The listing builds one solid part. Answer for the finished solid, in the listing's coordinates (mm). A direction names the side the tool comes from. Round coordinates to 2 decimals unless told otherwise and drop trailing zeros. Loops run counter-clockwise (first coordinate to the right, second up) from the corner with the lowest first, then second, coordinate; pieces in that order, holes last. Notation, with made-up numbers: (-33.75, -10) -> (9.25, -10) arc R19 ccw to (9.25, 10) -> close; hole circle Ø8 at (-5.5, -22.5). An arc over 180 degrees is marked (long way). One line per question, with ' | ' between items.
from build123d import *

# Parameters (mm, degrees)
F0_R     = 35
F0_R_2   = 25
F1_DEPTH = 100
F2_W     = 10
F2_H     = 8
F3_DEPTH = 100.001


with BuildPart() as f1:
    # F0 (on Front) → F1 (new body)
    with BuildSketch(Plane.XZ):
        Circle(F0_R)
        Circle(F0_R_2, mode=Mode.SUBTRACT)
    extrude(amount=F1_DEPTH)

    # F2 (on Front) → F3 (cut, through all)
    with BuildSketch(Plane.XZ):
        with Locations((0, 25)):
            Rectangle(F2_W, F2_H)
    extrude(amount=F3_DEPTH, mode=Mode.SUBTRACT)


solid = f1.part
Q1. A cutting plane is placed at B-B on z = 0. Give the vertices of the cut face in (x, y), plus the area to 3 significant figures.
Numbers:
outline: (-35, -100) -> (-25, -100) -> (-25, 0) -> (-35, 0) -> close; (25, -100) -> (35, -100) -> (35, 0) -> (25, 0) -> close | area: 2,000 mm^2
Q2. For faces 1 (the face through (-24, 0, 8)), 2 (the face through (-5, -49, 27)), determine the directions among +Z, -Z, +X, -X, +Y, -Y from which every point of the face is accessible in a straight line to the end or side of a thin tool.
Numbers:
face 1: +Z, -Z, +X, -X, +Y | face 2: +Y, -Y
Q3. Given pin 1 Ø12 at (x, y) = (-13.5, -54.5) entering from +Z; pin 2 Ø2 at (y, z) = (-25.5, 16) entering from +X; pin 3 Ø2 at (x, y) = (-4, -71.5) entering from -Z, each flat-ended and moving along its own axis, determine where each tip first touches the part or whether it passes through.
Numbers:
pin 1: z = 34.19 | pin 2: x = 31.62 | pin 3: z = -34.87
Q4. A cutting plane is placed at D-D on z = -28. Give the vertices of the cut face in (x, y), plus the area to 3 significant figures.
Numbers:
outline: (-21, -100) -> (21, -100) -> (21, 0) -> (-21, 0) -> close | area: 4,200 mm^2
Q5. A cutting plane is placed at A-A on x = 0. Give the vertices of the cut face in (y, z).
Numbers:
outline: (-100, -35) -> (0, -35) -> (0, -25) -> (-100, -25) -> close; (-100, 29) -> (0, 29) -> (0, 35) -> (-100, 35) -> close
Q6. For a pull along Z with two mould halves and no side action, classify faces 3 (the face through (-28, -49, -21)), 4 (the face through (5, -49, 27)), 5 (the face through (-24, -100, 8)) as pulls with the +Z half, pulls with the -Z half, needs draft (parallel to the pull), parting line crosses it, or undercut.
Numbers:
face 3: parting line crosses it | face 4: undercut | face 5: needs draft
Q7. A cutting plane is placed at C-C on y = -26. Give the vertices of the cut face in (x, z), plus the area to 3 significant figures.
Numbers:
outline: circle Ø70 at (0, 0); hole (-5, 24.49) arc R25 ccw (long way) to (5, 24.49) -> (5, 29) -> (-5, 29) -> close | area: 1,840 mm^2
Q8. Find the intervals of material crossed by line 1 (Z direction, x = 0, y = -52.5); line 2 (X direction, y = -64.5, z = 22); line 3 (X direction, y = -58, z = -16), in increasing order. Write a range as from..to.
Numbers:
line 1: -35..-25, 29..35 | line 2: -27.22..-11.87, 11.87..27.22 | line 3: -31.13..-19.21, 19.21..31.13
